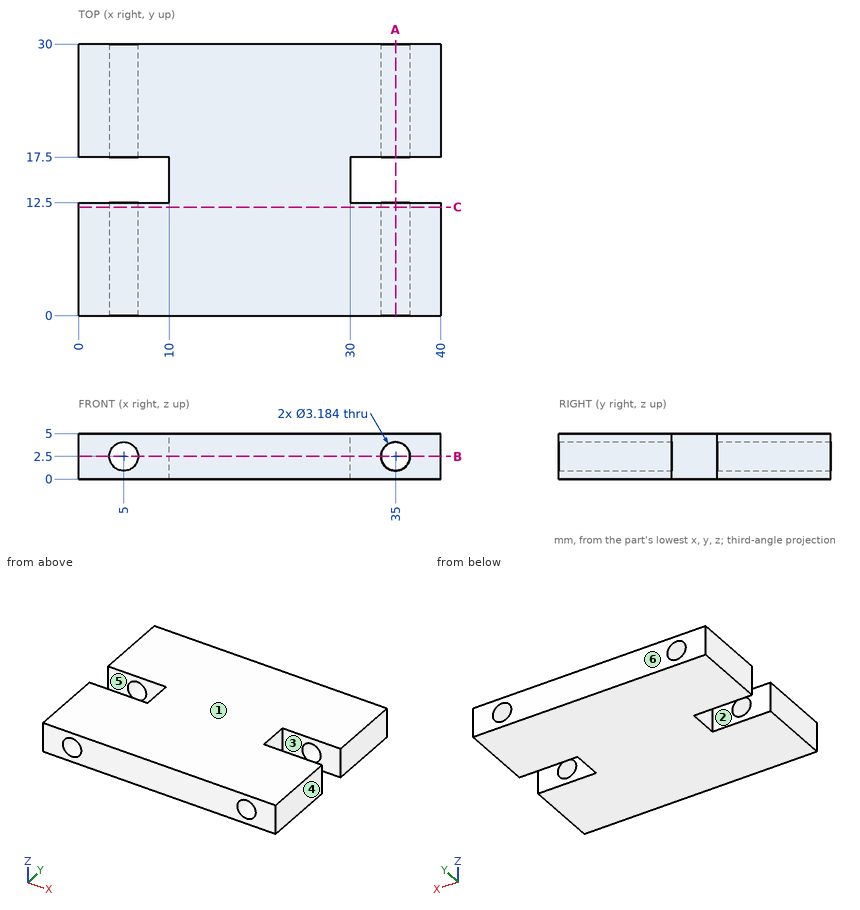
Design review of the part shown in the three views and the two pictorial views. Dimensions are in mm from the part's minimum x, y and z. A direction names the side the tool comes from. Coordinates: 2 decimals unless noted, no trailing zeros. Write each loop counter-clockwise with the first axis right and the second up, starting at its lowest first coordinate (ties: lowest second). Pieces come first, ordered by that corner, then holes.
1) Machinability: for the marked faces 1, 2 and 3, which of the approach directions +Z, -Z, +X, -X, +Y, -Y give a long, thin tool a straight path to every point of the face, cutting with its end or side? Answer none if there is none.
2) Clearance check with flat-ended pins moving along their axes: pin 1 Ø2.5 at (x, z) = (34, 1.5) entering from -Y; pin 2 Ø3 at (x, z) = (5, 2.5) entering from +Y. State where each tip first meets the part, or that it passes through.
3) We need section A-A on x = 35. State the section outline as (y, z) points.
4) We need section B-B on z = 2.5. State the section outline as (x, y) points, then the cut area to 3 significant figures.
5) The part is to be moulded in two halves that separate along Y. For the marked faces 4, 5 and 6, say which applies: pulls with the +Y half, pulls with the -Y half, needs draft (parallel to the pull), parting line crosses it, or undercut.
6) To check wall thickness, follow probe 1 along X at (y, z) = (8, 2.35) (1 decimal); probe 2 along X at (y, z) = (23, 2.95); probe 3 along Y at (x, z) = (31, 0.8). State the ranges of each line that lie inside material, in increasing order.
7) We need section C-C on y = 12. State the section outline as (x, z) points, then the cut area to 3 significant figures.
Answer list:
1. face 1: +Z, +X, -X, +Y, -Y
1. face 2: +Z, -Z, -X
1. face 3: +Z, -Z, +X
2. pin 1: stops at y = 0
2. pin 2: passes through
3. outline: (0, 0) - (12.5, 0) - (12.5, 0.91) - (0, 0.91) - close; (0, 4.09) - (12.5, 4.09) - (12.5, 5) - (0, 5) - close; (17.5, 0) - (30, 0) - (30, 0.91) - (17.5, 0.91) - close; (17.5, 4.09) - (30, 4.09) - (30, 5) - (17.5, 5) - close
4. outline: (0, 0) - (3.41, 0) - (3.41, 12.5) - (0, 12.5) - close; (0, 17.5) - (3.41, 17.5) - (3.41, 30) - (0, 30) - close; (6.59, 0) - (33.41, 0) - (33.41, 12.5) - (30, 12.5) - (30, 17.5) - (33.41, 17.5) - (33.41, 30) - (6.59, 30) - (6.59, 17.5) - (10, 17.5) - (10, 12.5) - (6.59, 12.5) - close; (36.59, 0) - (40, 0) - (40, 12.5) - (36.59, 12.5) - close; (36.59, 17.5) - (40, 17.5) - (40, 30) - (36.59, 30) - close
4. area: 941 mm2
5. face 4: needs draft
5. face 5: undercut
5. face 6: pulls with the +Y half
6. probe 1: x = 0 to 3.4, 6.6 to 33.4, 36.6 to 40
6. probe 2: x = 0 to 3.47, 6.53 to 33.47, 36.53 to 40
6. probe 3: y = 0 to 12.5, 17.5 to 30
7. outline: (0, 0) - (40, 0) - (40, 5) - (0, 5) - close; hole circle Ø3.18 at (5, 2.5); hole circle Ø3.18 at (35, 2.5)
7. area: 184 mm2
